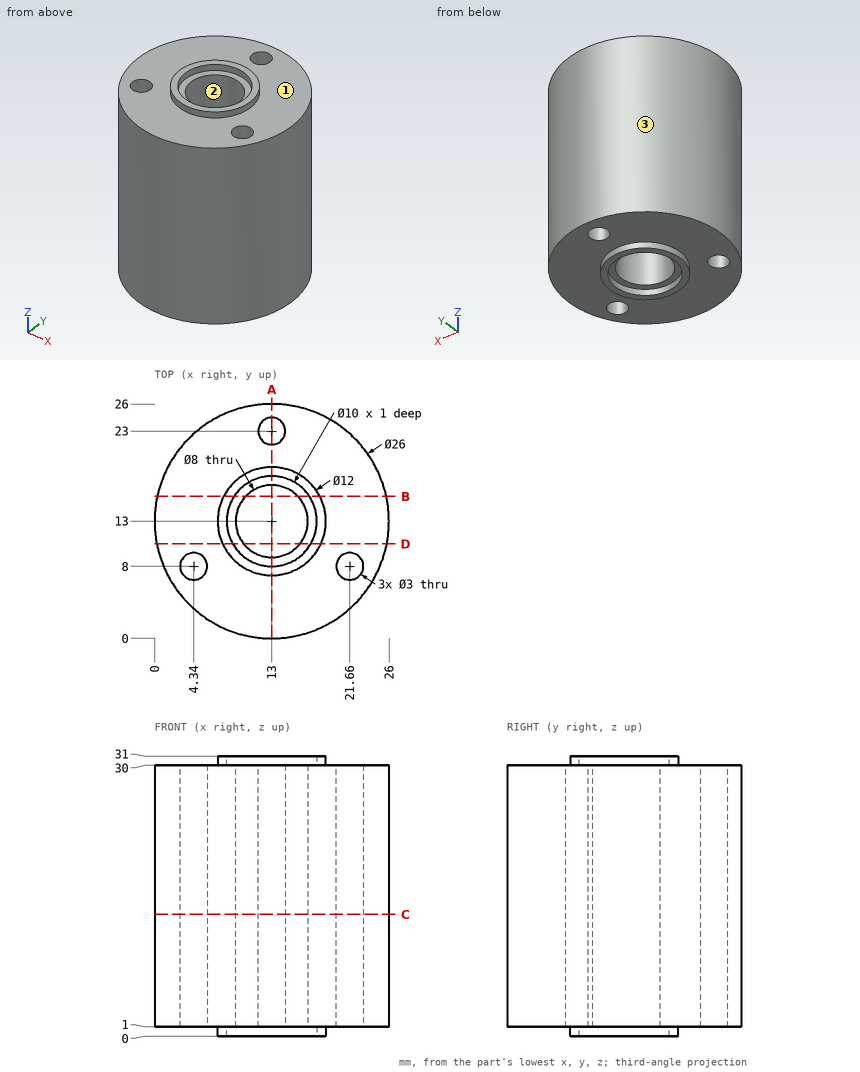
Could you check a few things on this drawing? It's one solid part, dimensions in mm from its lowest x, y, z. Coordinates: 2 decimals unless noted, no trailing zeros. Order: outer loops, then holes, each group sorted by start corner. A loop starts at its lowest first (then second) coordinate and runs counter-clockwise, first axis right, second up. Notation, with made-up numbers: (-9, -20) -> (18, -20) arc R25 cw to (18, 6) -> close; hole circle Ø5 at (-15.75, 83). An arc over 180 degrees is marked (long way). Answer in a Markdown table with one row per item.
(1) I want a section at B-B on y = 15.75. List the corners of the cut face in (x, z) for me (1 decimal).
Answer key:
| item | result |
|---|---|
| outline | (0.3, 1) -> (7.7, 1) -> (7.7, 0) -> (8.8, 0) -> (8.8, 1) -> (10.1, 1) -> (10.1, 30) -> (8.8, 30) -> (8.8, 31) -> (7.7, 31) -> (7.7, 30) -> (0.3, 30) -> close; (15.9, 1) -> (17.2, 1) -> (17.2, 0) -> (18.3, 0) -> (18.3, 1) -> (25.7, 1) -> (25.7, 30) -> (18.3, 30) -> (18.3, 31) -> (17.2, 31) -> (17.2, 30) -> (15.9, 30) -> close |
(2) Will these pins go through, and if not, where does the flat tip stop? pin 1 Ø1.5 at (x, y) = (19, 17) entering from +Z; pin 2 Ø12 at (y, z) = (6, 12) entering from -X; pin 3 Ø8 at (y, z) = (20, 17.5) entering from -X.
Answer key:
| item | result |
|---|---|
| pin 1 | z = 30 |
| pin 2 | x = 0.04 |
| pin 3 | x = 0.35 |
(3) I want a section at D-D on y = 10.5. List the corners of the cut face in (x, z) for me.
Answer key:
| item | result |
|---|---|
| outline | (0.24, 1) -> (7.55, 1) -> (7.55, 0) -> (8.67, 0) -> (8.67, 1) -> (9.88, 1) -> (9.88, 30) -> (8.67, 30) -> (8.67, 31) -> (7.55, 31) -> (7.55, 30) -> (0.24, 30) -> close; (16.12, 1) -> (17.33, 1) -> (17.33, 0) -> (18.45, 0) -> (18.45, 1) -> (25.76, 1) -> (25.76, 30) -> (18.45, 30) -> (18.45, 31) -> (17.33, 31) -> (17.33, 30) -> (16.12, 30) -> close |
(4) I want a section at C-C on z = 13.5. List the corners of the cut face in (x, y) for me.
Answer key:
| item | result |
|---|---|
| outline | circle Ø26 at (13, 13); hole circle Ø3 at (4.34, 8); hole circle Ø8 at (13, 13); hole circle Ø3 at (13, 23); hole circle Ø3 at (21.66, 8) |
(5) Thinking about a two-plate mould opening in Y: for the marked faces 1, 2 and 3, which applies, +Y half, -Y half, draft (parallel to the pull), parting line (faces both ways), or undercut?
Answer key:
| item | result |
|---|---|
| face 1 | draft |
| face 2 | undercut |
| face 3 | parting line |
(6) I want a section at A-A on x = 13. List the corners of the cut face in (y, z) for me, then the cut area to 3 significant figures.
Answer key:
| item | result |
|---|---|
| outline | (0, 1) -> (7, 1) -> (7, 0) -> (8, 0) -> (8, 1) -> (9, 1) -> (9, 30) -> (8, 30) -> (8, 31) -> (7, 31) -> (7, 30) -> (0, 30) -> close; (17, 1) -> (18, 1) -> (18, 0) -> (19, 0) -> (19, 1) -> (21.5, 1) -> (21.5, 30) -> (19, 30) -> (19, 31) -> (18, 31) -> (18, 30) -> (17, 30) -> close; (24.5, 1) -> (26, 1) -> (26, 30) -> (24.5, 30) -> close |
| area | 439 mm^2 |
(7) Please list where these lines run through material, in increasing order: probe 1 along Y at (x, z) = (13, 23.5); probe 2 along Y at (x, z) = (13, 0.6); probe 3 along X at (y, z) = (9.75, 29).
Answer key:
| item | result |
|---|---|
| probe 1 | 0 to 9, 17 to 21.5, 24.5 to 26 |
| probe 2 | 7 to 8, 18 to 19 |
| probe 3 | 0.41 to 10.67, 15.33 to 25.59 |
